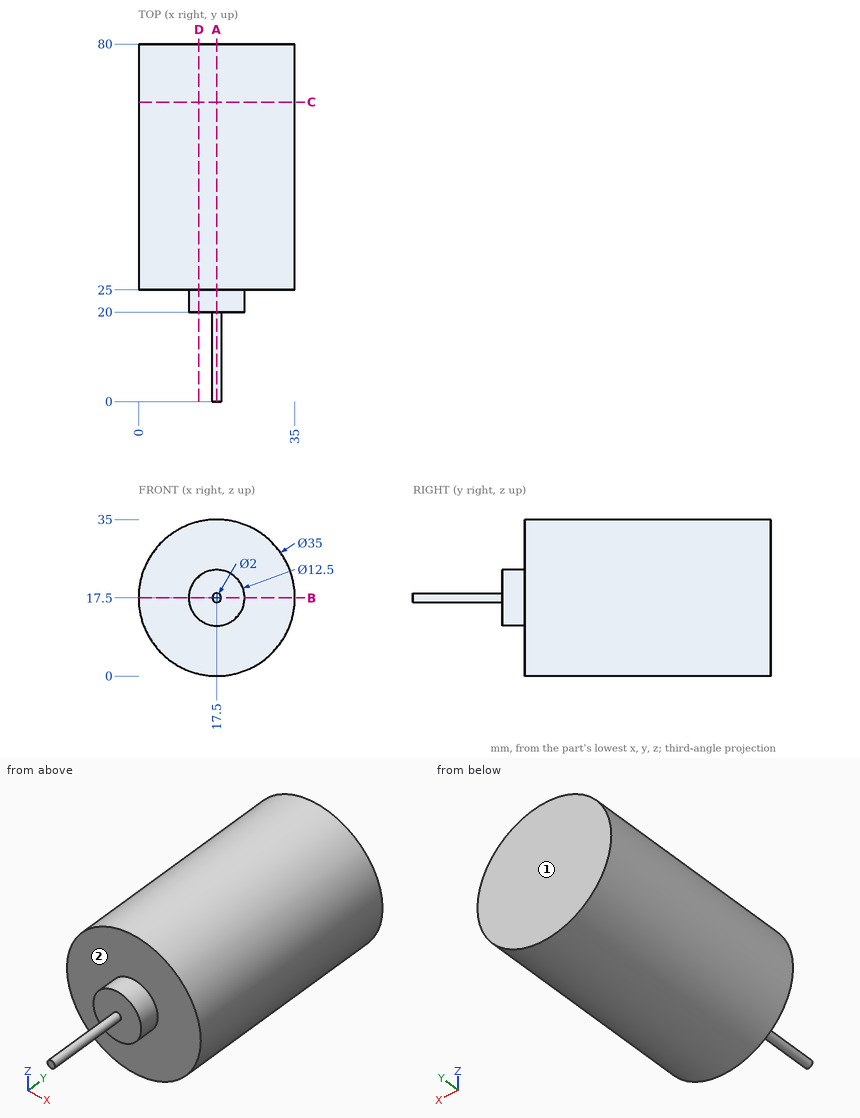
The figure shows three views and two pictorial views of one solid part (mm, origin at its lowest corner). Answer the questions. A direction names the side the tool comes from. Coordinates: 2 decimals unless noted, no trailing zeros. Loops run counter-clockwise (first coordinate to the right, second up) from the corner with the lowest first, then second, coordinate; pieces in that order, holes last.
(1) The part is cut by section D-D (x = 13.5). Determine the outline of the cut face in (y, z).
Solution:
outline: (20, 12.7) - (25, 12.7) - (25, 0.46) - (80, 0.46) - (80, 34.54) - (25, 34.54) - (25, 22.3) - (20, 22.3) - close
(2) A tool of negligible diameter and unlimited length cuts with its end or side. For the marked faces 1 and 2, from which of +Z, -Z, +X, -X, +Y, -Y can it reach the whole face along a straight path? Write none if from no direction.
Solution:
face 1: +Z, -Z, +X, -X, +Y
face 2: -Y
(3) Flat-ended cylindrical pins translate along their axes: pin 1 Ø6 at (y, z) = (20.5, 13.5) entering from -X; pin 2 Ø2 at (x, y) = (25, 44) entering from +Z; pin 3 Ø8 at (x, y) = (9, 70) entering from -Z; pin 4 Ø10.5 at (x, z) = (11.5, 17) entering from -Y. Find the tip coordinate at first contact, or state that the pin passes through.
Solution:
pin 1: stops at x = 11.33
pin 2: stops at z = 33.75
pin 3: stops at z = 0.59
pin 4: stops at y = 0
(4) The part is cut by section C-C (y = 67). Determine the outline of the cut face in (x, z), and give its area (3 significant figures).
Solution:
outline: circle Ø35 at (17.5, 17.5)
area: 962 mm2
(5) Consider line 1 along Y through (x, z) = (2.5, 12.5); line 2 along Z through (x, y) = (17, 45); line 3 along Y through (x, z) = (22, 14.5). Determine where each line is inside the solid, lowest interval first.
Solution:
line 1: y = 25 to 80
line 2: z = 0.01 to 34.99
line 3: y = 20 to 80
(6) The part is cut by section A-A (x = 17.5). Determine the outline of the cut face in (y, z).
Solution:
outline: (0, 16.5) - (20, 16.5) - (20, 11.25) - (25, 11.25) - (25, 0) - (80, 0) - (80, 35) - (25, 35) - (25, 23.75) - (20, 23.75) - (20, 18.5) - (0, 18.5) - close
(7) The part is cut by section B-B (z = 17.5). Determine the outline of the cut face in (x, y).
Solution:
outline: (0, 25) - (11.25, 25) - (11.25, 20) - (16.5, 20) - (16.5, 0) - (18.5, 0) - (18.5, 20) - (23.75, 20) - (23.75, 25) - (35, 25) - (35, 80) - (0, 80) - close
